```python
from build123d import *

# Parameters (mm, degrees)
BOSS_EXTRUDE3_DEPTH         = 19.05
F_1_4_0_25_DIAMETER_HOLE1_D = 6.35
F_6_32_TAPPED_HOLE1_REACH   = 166.777
F_6_32_TAPPED_HOLE1_BORE_R  = 1.35255


with BuildPart() as part:
    # Sketch1 → Boss-Extrude3 (new body)
    with BuildSketch(Plane(origin=(0, 0, 0), x_dir=(1, 0, 0), z_dir=(0, 1, 0))):
        with BuildLine():
            Line((63.73495, 0), (100.80625, 0))
            ThreePointArc((100.80625, 0), (113.59515, 12.7889), (126.38405, 0))
            Line((126.38405, 0), (162.56, 0))
            Line((162.56, 0), (162.56, 19.05))
            Line((162.56, 19.05), (0, 19.05))
            Line((0, 19.05), (0, 0))
            Line((0, 0), (36.17595, 0))
            ThreePointArc((36.17595, 0), (49.95545, 13.7795), (63.73495, 0))
        make_face()
    extrude(amount=BOSS_EXTRUDE3_DEPTH)

    # 1/4 (0.25) Diameter Hole1 (through all)
    with Locations(Plane.XY):
        with Locations((6.35, 9.525)):
            f_1_4_0_25_diameter_hole1 = Hole(F_1_4_0_25_DIAMETER_HOLE1_D / 2)

    # #6-32 Tapped Hole1 bore → #6-32 Tapped Hole1 (cut, up to next)
    with BuildSketch(Plane(origin=(0, 19.05, 0), x_dir=(1, 0, 0), z_dir=(0, 1, 0)), mode=Mode.PRIVATE) as f_6_32_tapped_hole1_sk1:
        with Locations((6.578923223, 9.508761569)):
            Circle(F_6_32_TAPPED_HOLE1_BORE_R)
    f_6_32_tapped_hole1_tool1 = extrude(f_6_32_tapped_hole1_sk1.sketch, amount=-F_6_32_TAPPED_HOLE1_REACH, mode=Mode.PRIVATE) & part.part
    f_6_32_tapped_hole1 = f_6_32_tapped_hole1_tool1.solids().sort_by_distance((6.578923, 19.05, -9.508762))[0]
    add(f_6_32_tapped_hole1, mode=Mode.SUBTRACT)

    # Mirror1: 1/4 (0.25) Diameter Hole1, #6-32 Tapped Hole1 across plane
    add(f_1_4_0_25_diameter_hole1.mirror(Plane.ZY.offset(-81.28)), mode=Mode.SUBTRACT)
    add(f_6_32_tapped_hole1.mirror(Plane.ZY.offset(-81.28)), mode=Mode.SUBTRACT)


solid = part.part
```
For this review, take the finished solid that the model builds, in its own axes (mm). A direction names the side the tool comes from. Coordinates: 2 decimals unless noted, no trailing zeros. Answer as CSV lines item,"result".
Q1. Wall thickness on line 1 along Y through (x, z) = (6.35, -6.25); line 2 along X through (y, z) = (2.5, -2.5); line 3 along X through (y, z) = (9.25, -1.25): over which ranges is each line inside the solid? List them lowest first. Write a range as [from, to].
Model answer:
line 1,"y = [0, 6.35], [12.7, 19.05]"
line 2,"x = [0, 36.4], [63.51, 101.05], [126.14, 162.56]"
line 3,"x = [0, 3.19], [9.51, 36.23], [63.68, 100.87], [126.32, 153.05], [159.37, 162.56]"
Q2. Clearance check with flat-ended pins moving along their axes: pin 1 Ø2 at (x, y) = (48, 13) entering from +Z; pin 2 Ø4 at (x, y) = (156.21, 9.525) entering from -Z. State where each tip first meets the part, or that it passes through.
Model answer:
pin 1,"stops at z = -13.46"
pin 2,"passes through"
Q3. Draft analysis for pull direction Y (two halves, no side actions). For faces 3 (the face through (4.9, 6.7, -9.7)), 4 (the face through (80, 0, -10)), 5 (the face through (113.314, 9.392, -12.786)), state which applies: released by +Y, released by -Y, zero draft, split by the parting line, or undercut.
Model answer:
face 3,"undercut"
face 4,"released by -Y"
face 5,"zero draft"
Q4. For faces 1 (the face through (5.228, 15.711, -9.568)), 2 (the face through (155.522, 6.426, -9.658)), list the 3-axis set-ups (+Z, -Z, +X, -X, +Y, -Y) from which the entire face can be reached by the end or side of a thin tool; tool diameter is ignored.
Model answer:
face 1,"+Y"
face 2,"+Z, -Z"
